```python
from build123d import *

# Parameters (mm, degrees)
F1_DEPTH = 9.551


with BuildPart() as f1:
    # F0 (on Front) → F1 (new body)
    with BuildSketch(Plane.XZ):
        with BuildLine():
            Line((0, -5), (0, 0))
            Line((0, 0), (0, 5.517102))
            Line((0, 5.517102), (-1.5, 5.517102))
            ThreePointArc((-1.5, 5.517102), (-2.207107, 5.224208), (-2.5, 4.517102))
            Line((-2.5, 4.517102), (-2.5, -4))
            ThreePointArc((-2.5, -4), (-2.207107, -4.707107), (-1.5, -5))
            Line((-1.5, -5), (0, -5))
        make_face()
    extrude(amount=F1_DEPTH)


solid = f1.part
```
Check sheet for the modelled part. Datum: model origin and axes. Units: mm. Round coordinates to 2 decimals unless told otherwise and drop trailing zeros. Write each loop counter-clockwise with the first axis right and the second up, starting at its lowest first coordinate (ties: lowest second). Pieces come first, ordered by that corner, then holes. Notation, with made-up numbers: (-6, -14) -> (26, -14) arc R18 cw to (26, -5) -> close; hole circle Ø5 at (47.5, 72). An arc over 180 degrees is marked (long way). One line per question, with ' | ' between items. Start each with the question number.
1. Sectioned sample at B-B, the plane x = -2.25. Record the cut outline in (y, z).
2. Release check for a two-part mould opening along Y. For faces 1 (the face through (-2.5, -5, 0)), 2 (the face through (-1, 0, 0)), 3 (the face through (-1, -9.551, 0)) record: +Y half, -Y half, draft (parallel to the pull), parting line (faces both ways), or undercut.
3. Sectioned sample at A-A, the plane y = -5. Record the cut outline in (x, z).
4. Scan lines: line 1 along Z through (x, y) = (-2.2, -6.25); line 2 along Z through (x, y) = (-2.4, -1.25). Record each from-to range of solid material in increasing order. Write a range as from..to.
Taken from the geometry:
1) outline: (-9.55, -4.66) -> (0, -4.66) -> (0, 5.18) -> (-9.55, 5.18) -> close
2) face 1: draft | face 2: +Y half | face 3: -Y half
3) outline: (-2.5, -4) arc R1 ccw to (-1.5, -5) -> (0, -5) -> (0, 5.52) -> (-1.5, 5.52) arc R1 ccw to (-2.5, 4.52) -> close
4) line 1: z = -4.71..5.23 | line 2: z = -4.44..4.95
